```python
from build123d import *

# Parameters (mm, degrees)
SKETCH1_R           = 50
BOSS_EXTRUDE1_DEPTH = 4
SKETCH2_R           = 4
CUT_EXTRUDE1_DEPTH  = 4
CIRPATTERN1_COUNT   = 16
CUT_EXTRUDE2_DEPTH  = 4
CIRPATTERN3_COUNT   = 6
SKETCH5_R           = 1.9
CUT_EXTRUDE3_DEPTH  = 4


with BuildPart() as part:
    # Sketch1 → Boss-Extrude1 (new body)
    with BuildSketch(Plane(origin=(0, 0, 0), x_dir=(1, 0, 0), z_dir=(0, 1, 0))):
        with Locations(Location((0, 0, 0), (0, 0, 270))):
            Circle(SKETCH1_R)
    extrude(amount=BOSS_EXTRUDE1_DEPTH)

    # Sketch2 → Cut-Extrude1 (cut)
    with BuildSketch(Plane(origin=(0, 4, 0), x_dir=(1, 0, 0), z_dir=(0, 1, 0))):
        with Locations(Location((0, 43, 0), (0, 0, 270))):
            Circle(SKETCH2_R)
    cut_extrude1 = extrude(amount=-CUT_EXTRUDE1_DEPTH, mode=Mode.SUBTRACT)

    # CirPattern1: Cut-Extrude1 ×16 about axis
    cirpattern1_axis = Axis((0, 0, 0), (0, 1, 0))
    for i in range(1, CIRPATTERN1_COUNT):
        add(cut_extrude1.rotate(cirpattern1_axis, i * 360 / CIRPATTERN1_COUNT), mode=Mode.SUBTRACT)

    # Sketch3 → Cut-Extrude2 (cut)
    with BuildSketch(Plane(origin=(0, 4, 0), x_dir=(1, 0, 0), z_dir=(0, 1, 0))):
        with BuildLine():
            Line((2.124355653, 17.320508076), (10, 17.320508076))
            Line((10, 17.320508076), (26.001479795, 17.320508076))
            ThreePointArc((26.001479795, 17.320508076), (28.697954971, 19.005585406), (28.365250686, 22.167826992))
            ThreePointArc((28.365250686, 22.167826992), (19.971239607, 29.952455468), (9.557608221, 34.70809884))
            ThreePointArc((9.557608221, 34.70809884), (7.622675946, 34.591346868), (6.163064658, 33.31575727))
            Line((6.163064658, 33.31575727), (-0.473720558, 21.820508076))
            ThreePointArc((-0.473720558, 21.820508076), (-0.473720558, 18.820508076), (2.124355653, 17.320508076))
        make_face()
    cut_extrude2 = extrude(amount=-CUT_EXTRUDE2_DEPTH, mode=Mode.SUBTRACT)

    # CirPattern3: Cut-Extrude2 ×6 about axis
    cirpattern3_axis = Axis((0, 0, 0), (0, 1, 0))
    for i in range(1, CIRPATTERN3_COUNT):
        add(cut_extrude2.rotate(cirpattern3_axis, i * 360 / CIRPATTERN3_COUNT), mode=Mode.SUBTRACT)

    # Sketch5 → Cut-Extrude3 (cut)
    with BuildSketch(Plane(origin=(0, 4, 0), x_dir=(1, 0, 0), z_dir=(0, 1, 0))):
        with Locations(Location((0, 9.95, 0), (0, 0, 270))):
            Circle(SKETCH5_R)
        with Locations(Location((0, 0, 0), (0, 0, 270))):
            Circle(SKETCH5_R)
        with Locations(Location((0, -9.95, 0), (0, 0, 270))):
            Circle(SKETCH5_R)
    extrude(amount=-CUT_EXTRUDE3_DEPTH, mode=Mode.SUBTRACT)


solid = part.part
```
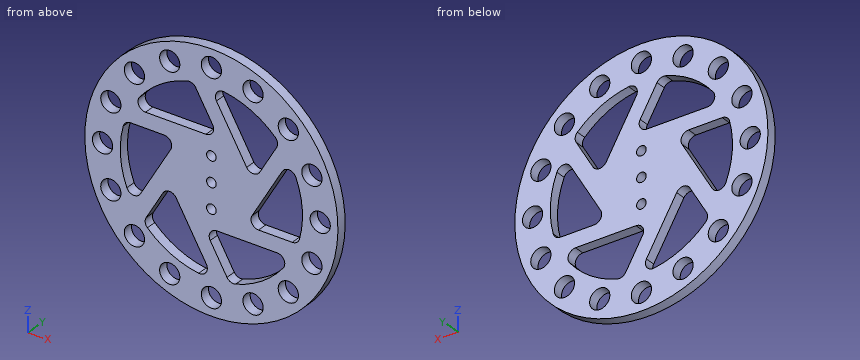
Source: CAD feature listing. Evaluate the final solid. Frame: model axes, mm. Give positions to 0.01 mm unless a question says otherwise; leave off trailing zeros. Order: outer loops, then holes, each group sorted by start corner. A loop starts at its lowest first (then second) coordinate and runs counter-clockwise, first axis right, second up. Notation, with made-up numbers: (44.25, 65.25) -> (61.25, 65.25) arc R16 ccw to (61.25, 77.25) -> close; hole circle Ø10 at (-37.75, 86). An arc over 180 degrees is marked (long way). Use a Markdown table: item, result.
Q1. Section A-A (z = 0). Return the cut outline in (x, y), and give its area (3 significant figures).
A:
| item | result |
|---|---|
| outline | (-50, 0) -> (-47, 0) -> (-47, 4) -> (-50, 4) -> close; (-39, 0) -> (-36, 0) -> (-36, 4) -> (-39, 4) -> close; (-20, 0) -> (-1.9, 0) -> (-1.9, 4) -> (-20, 4) -> close; (1.9, 0) -> (20, 0) -> (20, 4) -> (1.9, 4) -> close; (36, 0) -> (39, 0) -> (39, 4) -> (36, 4) -> close; (47, 0) -> (50, 0) -> (50, 4) -> (47, 4) -> close |
| area | 193 mm^2 |
Q2. Material intervals for line 1 (Z direction, x = -3.5, y = 0.2); line 2 (X direction, y = 2.6, z = 25.5); line 3 (X direction, y = 3.3, z = -13), sorted ascending. Write a range as [from, to].
A:
| item | result |
|---|---|
| line 1 | [-49.88, -44.94], [-41.06, -35.47], [-28.58, 17.32], [28.7, 41.06], [44.94, 49.88] |
| line 2 | [-43.01, -25.41], [-1.65, 5.28], [25.4, 43.01] |
| line 3 | [-48.28, -41.74], [-37.71, -33.57], [-27.51, -20.58], [-12.49, 37.71], [41.74, 48.28] |
Q3. Section B-B (x = -41.5). Return the cut outline in (y, z).
A:
| item | result |
|---|---|
| outline | (0, -27.89) -> (4, -27.89) -> (4, -20.04) -> (0, -20.04) -> close; (0, -12.87) -> (4, -12.87) -> (4, -3.71) -> (0, -3.71) -> close; (0, 3.71) -> (4, 3.71) -> (4, 12.87) -> (0, 12.87) -> close; (0, 20.04) -> (4, 20.04) -> (4, 27.89) -> (0, 27.89) -> close |
Q4. Section C-C (y = 2). State how many separate pieces and enclosed holes the cut face has, and give its area (3 significant figures).
A:
| item | result |
|---|---|
| separate pieces | 1 |
| enclosed holes | 25 |
| area | 4,840 mm^2 |
Q5. First-contact query: P1, Ø2, axis at x = 16.5, y = 2.5, coming from the -Z side; P2, Ø1.5, axis at x = 7.5, y = 1.5, coming from the -Z side. Flat tips, straight axial feed; report the tip coordinate or a pass-through.
A:
| item | result |
|---|---|
| P1 | z = -47.54 |
| P2 | z = -49.54 |
